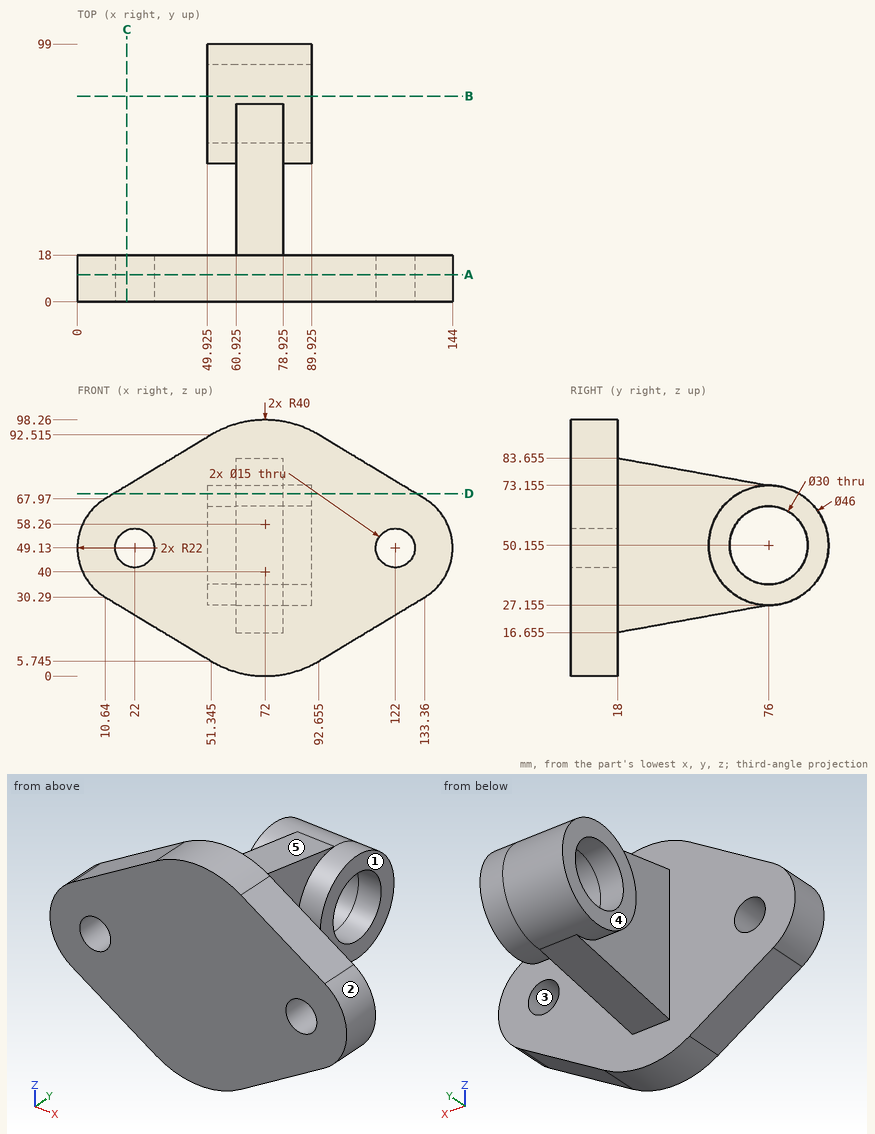
Geometry check sheet. Reference: drawing and pictorial views, mm from the part's lowest x, y, z. A direction names the side the tool comes from. Coordinates: 2 decimals unless noted, no trailing zeros. Order: outer loops, then holes, each group sorted by start corner. A loop starts at its lowest first (then second) coordinate and runs counter-clockwise, first axis right, second up. Notation, with made-up numbers: (68, 27.25) -> (118, 27.25) arc R21 ccw to (118, 61.25) -> close; hole circle Ø6 at (35, 61.5). An arc over 180 degrees is marked (long way). Write item = value, one per line. Start each with the question number.
1) Cross-section at A-A (y = 10.5). Enter the section's corners in (x, z) (1 decimal).
2) Cross-section at B-B (y = 79). Enter the section's corners in (x, z) (1 decimal).
3) Cross-section at C-C (x = 19). Enter the section's corners in (y, z).
4) Go/stop test with flat-tipped pins: P1, Ø17.5, axis at y = 59, z = 38, coming from the +X side (1 decimal); P2, Ø17.5, axis at y = 49, z = 66, coming from the -X side (1 decimal); P3, Ø12, axis at x = 80, y = 87, coming from the -Z side (1 decimal); P4, Ø1, axis at x = 46.5, z = 78.5, coming from the -Y side. Record where each tip stops, or that it passes through.
5) Access from +Z, -Z, +X, -X, +Y, -Y to the whole of each face (thin tool, end or side, straight path). Record for the marked faces 1 and 2.
6) Cross-section at D-D (z = 70). Enter the section's corners in (x, y) (1 decimal), then the cut area to 3 significant figures.
7) Material ranges on L1, parallel to Z at x = 58.25, y = 76 (1 decimal); L2, parallel to Y at x = 82, z = 48 (1 decimal); L3, parallel to Y at x = 108.5, z = 66, recorded low to high.
8) Mould release check, pull along Z, two halves, no side actions. Record for the marked faces 3, 4 and 5: +Z half, -Z half, draft (parallel to the pull), parting line (faces both ways), or undercut.
Ans:
q1.outline = (10.6, 30.3) -> (51.3, 5.7) arc R40 ccw to (92.7, 5.7) -> (133.4, 30.3) arc R22 ccw to (133.4, 68) -> (92.7, 92.5) arc R40 ccw to (51.3, 92.5) -> (10.6, 68) arc R22 ccw to start; hole circle Ø15 at (22, 49.1); hole circle Ø15 at (122, 49.1)
q2.outline = (49.9, 27.4) -> (89.9, 27.4) -> (89.9, 35.5) -> (49.9, 35.5) -> close; (49.9, 64.9) -> (89.9, 64.9) -> (89.9, 73) -> (49.9, 73) -> close
q3.outline = (0, 25.25) -> (18, 25.25) -> (18, 42.26) -> (0, 42.26) -> close; (0, 56) -> (18, 56) -> (18, 73.01) -> (0, 73.01) -> close
q4.P1 = 89.9
q4.P2 = 49.9
q4.P3 = 27.7
q4.P4 = 0
q5.face_1 = +Z, -Z, +X, +Y
q5.face_2 = +X, +Y, -Y
q6.outline = (14, 0) -> (130, 0) -> (130, 18) -> (78.9, 18) -> (78.9, 64.4) -> (89.9, 64.4) -> (89.9, 87.6) -> (49.9, 87.6) -> (49.9, 64.4) -> (60.9, 64.4) -> (60.9, 18) -> (14, 18) -> close
q6.area = 3,850 mm²
q7.L1 = 27.2 to 35.2, 65.2 to 73.2
q7.L2 = 0 to 18, 53.1 to 61.2, 90.8 to 98.9
q7.L3 = 0 to 18
q8.face_3 = undercut
q8.face_4 = draft
q8.face_5 = +Z half
